```python
from build123d import *

# Parameters (mm, degrees)
F0_W     = 1270
F0_H     = 508
F1_DEPTH = 25.4
F2_W     = 1117.6
F2_H     = 355.6
F3_DEPTH = 101.6
F4_W     = 76.2
F4_H     = 76.2
F5_DEPTH = 288.925
F6_W     = 355.6
F6_H     = 19.05
F7_DEPTH = 965.2


with BuildPart() as f1:
    # F0 (on Top) → F1 (new body)
    with BuildSketch(Plane.XY):
        Rectangle(F0_W, F0_H)
    extrude(amount=F1_DEPTH)

    # F2 (on face) → F3 (join)
    with BuildSketch(Plane(origin=(0, 0, 0), x_dir=(1, 0, 0), z_dir=(0, 0, -1))):
        Rectangle(F2_W, F2_H)
    extrude(amount=F3_DEPTH)

    # F4 (on face) → F5 (join)
    with BuildSketch(Plane(origin=(0, 0, -101.6), x_dir=(1, 0, 0), z_dir=(0, 0, -1))):
        with Locations((-520.7, 139.7)):
            Rectangle(F4_W, F4_H)
        with Locations((-520.7, -139.7)):
            Rectangle(F4_W, F4_H)
        with Locations((520.7, 139.7)):
            Rectangle(F4_W, F4_H)
        with Locations((520.7, -139.7)):
            Rectangle(F4_W, F4_H)
    extrude(amount=F5_DEPTH)

    # F6 (on face) → F7 (join, through all)
    with BuildSketch(Plane.YZ.offset(-482.6)):
        with Locations((0, -267.423869)):
            Rectangle(F6_W, F6_H)
    extrude(amount=F7_DEPTH)


solid = f1.part
```
Geometry check sheet. Reference: the model listing, model coordinates, mm. A direction names the side the tool comes from. Coordinates: 2 decimals unless noted, no trailing zeros. Loops run counter-clockwise (first coordinate to the right, second up) from the corner with the lowest first, then second, coordinate; pieces in that order, holes last. Notation, with made-up numbers: (74, 29) -> (116, 29) arc R5 ccw to (116, 36) -> close; hole circle Ø9 at (-22, -33.5). An arc over 180 degrees is marked (long way). Put each result on its own line as item: value.
1) Cross-section at B-B on x = -154. Record the boundary of the cut face in (y, z), plus the area to 3 significant figures.
Result set:
outline: (-254, 0) -> (-177.8, 0) -> (-177.8, -101.6) -> (177.8, -101.6) -> (177.8, 0) -> (254, 0) -> (254, 25.4) -> (-254, 25.4) -> close; (-177.8, -276.95) -> (177.8, -276.95) -> (177.8, -257.9) -> (-177.8, -257.9) -> close
area: 55,800 mm^2
2) Cross-section at C-C on z = -305. Record the boundary of the cut face in (x, y).
Result set:
outline: (-558.8, -177.8) -> (-482.6, -177.8) -> (-482.6, -101.6) -> (-558.8, -101.6) -> close; (-558.8, 101.6) -> (-482.6, 101.6) -> (-482.6, 177.8) -> (-558.8, 177.8) -> close; (482.6, -177.8) -> (558.8, -177.8) -> (558.8, -101.6) -> (482.6, -101.6) -> close; (482.6, 101.6) -> (558.8, 101.6) -> (558.8, 177.8) -> (482.6, 177.8) -> close
3) Tool access check on faces 5 (the flat face through (482.6, -139, -333)), 6 (the flat face through (-482.6, 140, -179)), 7 (the flat face through (-8, -2, -101.6)), 8 (the flat face through (558.8, 2, -62)), 9 (the flat face through (-50, -187, 0)). Record the directions out of +Z, -Z, +X, -X, +Y, -Y that give a thin tool (end or side, any length) a straight path to the whole face; none if there is none.
Result set:
face 5: -Z, +Y, -Y
face 6: +Y, -Y
face 7: none
face 8: -Z, +X, +Y, -Y
face 9: -Z
4) Cross-section at D-D on y = -141.5. Record the boundary of the cut face in (x, z) (3 decimals), plus the area to 3 significant figures.
Result set:
outline: (-635, 0) -> (-558.8, 0) -> (-558.8, -390.525) -> (-482.6, -390.525) -> (-482.6, -276.949) -> (482.6, -276.949) -> (482.6, -390.525) -> (558.8, -390.525) -> (558.8, 0) -> (635, 0) -> (635, 25.4) -> (-635, 25.4) -> close; hole (-482.6, -257.899) -> (482.6, -257.899) -> (482.6, -101.6) -> (-482.6, -101.6) -> close
area: 208,000 mm^2
5) Thickness scan on line 1 (Z direction, x = 253.5, y = 141.5); line 2 (X direction, y = 140, z = -325.5); line 3 (Y direction, x = 502, z = -99.5). Record the ranges inside material, lowest first.
Result set:
line 1: z = -276.95 to -257.9, -101.6 to 25.4
line 2: x = -558.8 to -482.6, 482.6 to 558.8
line 3: y = -177.8 to 177.8
6) Cross-section at A-A on y = -54. Record the boundary of the cut face in (x, z), plus the area to 3 significant figures.
Result set:
outline: (-635, 0) -> (-558.8, 0) -> (-558.8, -101.6) -> (558.8, -101.6) -> (558.8, 0) -> (635, 0) -> (635, 25.4) -> (-635, 25.4) -> close; (-482.6, -276.95) -> (482.6, -276.95) -> (482.6, -257.9) -> (-482.6, -257.9) -> close
area: 164,000 mm^2
7) Release check for a two-part mould opening along Y. For faces 1 (the flat face through (-9, 254, 13)), 2 (the flat face through (-8, -177.8, -68)), 3 (the flat face through (520, 101.6, -244)), 4 (the flat face through (-482.6, 140, -333)) record: released by +Y, released by -Y, zero draft, split by the parting line, or undercut.
Result set:
face 1: released by +Y
face 2: released by -Y
face 3: undercut
face 4: zero draft
8) Gauge pin test, flat ends, axial feed: pin 1 Ø23 at (x, z) = (-526, -198.5) entering from -Y; pin 2 Ø2 at (y, z) = (56, -30.5) entering from -X; pin 3 Ø1.5 at (y, z) = (-3.5, -94) entering from +X; pin 4 Ø12 at (y, z) = (37.5, -113) entering from +X. Record the tip position at first contact, or that the pin passes through.
Result set:
pin 1: stops at y = -177.8
pin 2: stops at x = -558.8
pin 3: stops at x = 558.8
pin 4: passes through
